Here's how the part is built. I have some questions about the finished solid (model axes, mm). Face numbers are marked on the shaded views. A direction names the side the tool comes from. Coordinates: 2 decimals unless noted, no trailing zeros. Loops run counter-clockwise (first coordinate to the right, second up) from the corner with the lowest first, then second, coordinate; pieces in that order, holes last. Notation, with made-up numbers: (29.5, -39) -> (56.5, -39) arc R6 ccw to (56.5, -34) -> close; hole circle Ø10 at (31.5, 74.25). An arc over 180 degrees is marked (long way). Answer as a JSON object with one key per item and string values. Group by question number.
Q1. I want a section at C-C on x = -162. Write out the boundary of the cut face in (y, z).
Q2. I want a section at B-B on y = 715. Write out the boundary of the cut face in (x, z), then the cut area to 3 significant figures.
Q3. I want a section at A-A on z = 18. Write out the boundary of the cut face in (x, y), then the cut area to 3 significant figures.
Q4. I'm going to push flat-ended pins straight in: pin 1 (5 mm diameter, centred on y = 663, z = 58, fed in from +X); pin 2 (6 mm diameter, centred on y = 684.5, z = 35.5, fed in from +X); pin 3 (4 mm diameter, centred on x = -353.5, z = 50.5, fed in from -Y). Where does each tip first touch, or does it pass through?
Q5. On a 3-axis mill with a long thin cutter (end or side, diameter ignored), from which of +Z, -Z, +X, -X, +Y, -Y can I reach the whole of each face in a straight line? I mean the marked faces 1 and 2. Say none if no direction works.
Q6. I need wall thicknesses on line 1 (Y direction, x = -72, z = 31.5); line 2 (Y direction, x = -362, z = 14.5); line 3 (X direction, y = 663, z = 74.5). Which ranges of each line are inside material? Lowest first, please.
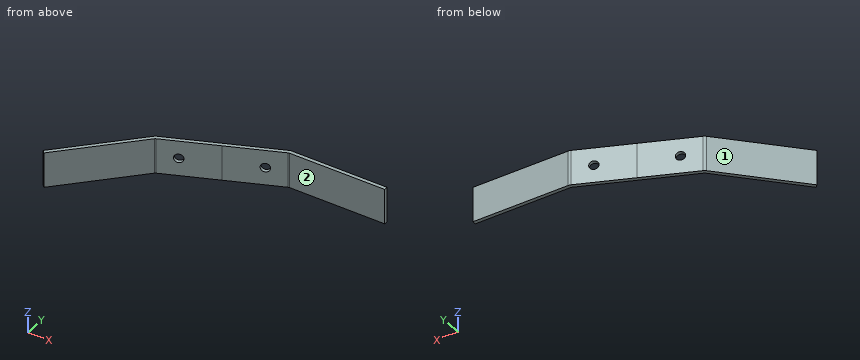
Autodesk Inventor part; units mm, degrees
ref_plane "YZ Plane" through (0, 0, 0) normal (1, 0, 0) x (0, 1, 0)
ref_plane "XZ Plane" through (0, 0, 0) normal (0, 1, 0) x (-1, 0, 0)
ref_plane "XY Plane" through (0, 0, 0) normal (0, 0, 1) x (1, 0, 0)
sketch "Sketch2" plane through (0, 0, 0) normal (0, 0, 1) x (1, 0, 0)
  line L0 (0, 277.6336) -> (196.3166, 196.3166) construction
  line L1 (196.3166, 196.3166) -> (277.6336, 0) construction
  line L2 (277.6336, 0) -> (196.3166, -196.3166) construction
  line L3 (196.3166, -196.3166) -> (0, -277.6336) construction
  line L4 (0, -277.6336) -> (-196.3166, -196.3166) construction
  line L5 (-196.3166, -196.3166) -> (-277.6336, 0) construction
  line L6 (-277.6336, 0) -> (-196.3166, 196.3166) construction
  line L7 (-196.3166, 196.3166) -> (0, 277.6336) construction
  line L8 (-196.3166, 196.3166) -> (0, 277.6336) construction
  line L9 (-461.2666, 773.8898) -> (-221.0579, 873.3874) construction
  line L10 (-98.1583, 236.9751) -> (-341.1623, 823.6386) construction
  line L11 (-221.0579, 873.3874) -> (0, 873.3874) construction
  line L12 (0, 873.3874) -> (0, 277.6336) construction
  line L13 (-461.2666, 773.8898) -> (-617.5782, 617.5782) construction
  line L14 (-617.5782, 617.5782) -> (-196.3166, 196.3166) construction
  line L15 (-223.0037, 867.1695) -> (-339.2489, 819.0192)
  line L16 (-5, 868.3874) -> (-216.8808, 868.3874)
  line L17 (-455.494, 770.8689) -> (-339.2489, 819.0192)
  line L18 (-610.5071, 617.5782) -> (-460.6848, 767.4005)
  arc A0 (-216.8808, 868.3874) -> (-223.0037, 867.1695) centre (-216.8808, 852.3874) ccw
  arc A1 (-455.494, 770.8689) -> (-460.6848, 767.4005) centre (-449.3711, 756.0868) ccw
  point P0 (0, 0)
  point P1 (0, 0)
  point P2 (0, 0)
  point P3 (-220.0634, 868.3874)
  point P4 (-458.4343, 769.651)
  dimension "d0" = 513
  dimension "d1" = 260
  dimension "d2" = 635
  dimension "d6" = 5
  dimension "d10" = 5
  dimension "d14" = 5
  dimension "d15" = 16
contour flange "Contour Flange1" sketch "Sketch2" thickness 8 bend radius 8 width 80 along (0, 0, 1) mid plane no both sides no wall seen from (-110.9404, 868.3874, 0) lies toward (0, -1, 0) curves L16 A0 L15 L17 A1 L18
bend "Bend1"
corner "Corner1"
sketch "Sketch3" plane through (-455.494, 770.8689, 80) normal (-0.3826834, 0.9238795, 0) x (0.9238795, 0.3826834, 0)
  line L0 (125.8228, 80) -> (125.8228, 0) construction
  line L1 (0, 0) -> (251.6457, 0)
  circle A0 centre (43.3228, 40) radius 10
  circle A1 centre (208.3228, 40) radius 10
  point P0 (125.8228, 40)
  dimension "d27" = 20
  dimension "d28" = 82.5
extrude "Extrusion1" cut sketch "Sketch3" against normal up to surface (8 mm away)
equation "\"d0\" = Барабан_габарит_по_кассетам"
equation "\"d1\" = Кассета_длина_грани"
equation "\"d2\" = Кассета_высота"
equation "\"d10\" = d6"
equation "\"d15\" = BendRadius + Thickness"
equation "\"d16\" = Thickness"
equation "\"d17\" = BendReliefWidth"
equation "\"d18\" = BendReliefDepth"
equation "\"d19\" = MinimumRemnant"
equation "\"d20\" = TransitionRadius"
equation "\"d22\" = BendRadius"
equation "\"d24\" = CornerReliefSize"
equation "\"d25\" = GapSize"
equation "\"d26\" = JacobiRadiusSize"
equation "\"BendRadius\" = Thickness"
equation "\"BendReliefWidth\" = Thickness"
equation "\"BendReliefDepth\" = 0.5 * Thickness"
equation "\"CornerReliefSize\" = 4 * Thickness"
equation "\"MinimumRemnant\" = 2 * Thickness"
equation "\"TransitionRadius\" = BendRadius"
equation "\"JacobiRadiusSize\" = BendRadius"
equation "\"GapSize\" = Thickness"
properties part number "ДМФ 01 52 Верхний лист"
Result set:
{
 "1": {"outline": "(860.39, 0) -> (868.39, 0) -> (868.39, 80) -> (860.39, 80) -> close"},
 "2": {"outline": "(-513.09, 0) -> (-501.77, 0) -> (-501.77, 80) -> (-513.09, 80) -> close", "area": "905 mm²"},
 "3": {"outline": "(-610.51, 617.58) -> (-604.85, 611.92) -> (-455.03, 761.74) arc R8 cw to (-452.43, 763.48) -> (-336.19, 811.63) -> (-219.94, 859.78) arc R8 cw to (-216.88, 860.39) -> (-5, 860.39) -> (-5, 868.39) -> (-216.88, 868.39) arc R16 ccw to (-223, 867.17) -> (-339.25, 819.02) -> (-455.49, 770.87) arc R16 ccw to (-460.68, 767.4) -> close", "area": "5,480 mm²"},
 "4": {"pin 1": "stops at x = -551.27", "pin 2": "stops at x = -529.27", "pin 3": "stops at y = 803.63"},
 "5": {"face 1": "+Z, -Z, -X, +Y", "face 2": "+Z, -Z, +X, -Y"},
 "6": {"line 1": "y = 860.39 to 868.39", "line 2": "y = 800.94 to 809.6", "line 3": "x = -565.09 to -553.77"}
}
